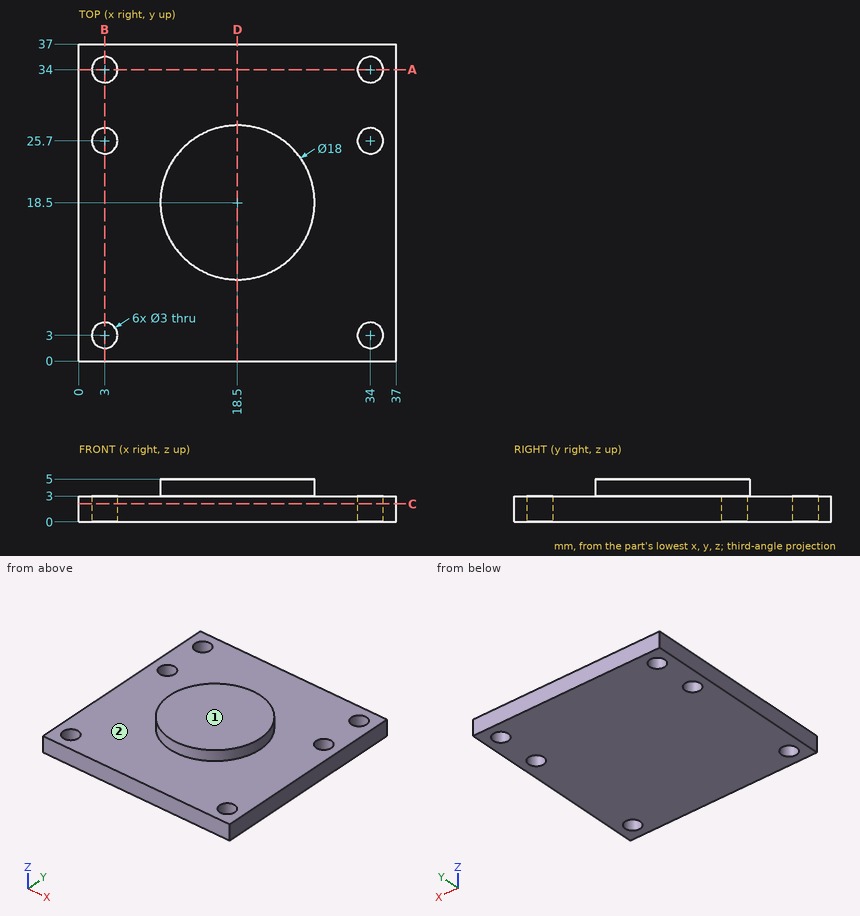
The drawing under review shows one solid part. Ordinate dimensions are in mm from its lowest x, y, z. A direction names the side the tool comes from. Round coordinates to 2 decimals unless told otherwise and drop trailing zeros. Loops run counter-clockwise (first coordinate to the right, second up) from the corner with the lowest first, then second, coordinate; pieces in that order, holes last. Notation, with made-up numbers: (21.25, 53) - (28.25, 53) arc R31 ccw to (28.25, 86) - close; hole circle Ø8 at (36.25, 5). An arc over 180 degrees is marked (long way). One line per item, written item: value. Start each with the question number.
1) Consider section C-C on z = 2.1. Give the boundary of the cut face in (x, y).
2) Consider section D-D on x = 18.5. Give the boundary of the cut face in (y, z).
3) Consider section B-B on x = 3. Give the boundary of the cut face in (y, z).
4) For the marked faces 1 and 2, list the 3-axis set-ups (+Z, -Z, +X, -X, +Y, -Y) from which the entire face can be reached by the end or side of a thin tool; tool diameter is ignored.
5) Insertion check: pin 1 Ø5 at (x, y) = (34, 25.7) entering from +Z; pin 2 Ø2 at (y, z) = (10.5, 4.5) entering from -X. Each pin has a flat end and moves straight along its axis. Give the tip position at first contact, or say it passes through.
6) To check wall thickness, follow L1, parallel to Y at x = 3, z = 1.6; L2, parallel to Z at x = 7.5, y = 32; L3, parallel to Y at x = 16.5, z = 3.05. State the ranges of each line that lie inside material, in increasing order. Write a range as from..to.
7) Consider section A-A on y = 34. Give the boundary of the cut face in (x, z).
Reported:
1. outline: (0, 0) - (37, 0) - (37, 37) - (0, 37) - close; hole circle Ø3 at (3, 3); hole circle Ø3 at (3, 25.7); hole circle Ø3 at (3, 34); hole circle Ø3 at (34, 3); hole circle Ø3 at (34, 25.7); hole circle Ø3 at (34, 34)
2. outline: (0, 0) - (37, 0) - (37, 3) - (27.5, 3) - (27.5, 5) - (9.5, 5) - (9.5, 3) - (0, 3) - close
3. outline: (0, 0) - (1.5, 0) - (1.5, 3) - (0, 3) - close; (4.5, 0) - (24.2, 0) - (24.2, 3) - (4.5, 3) - close; (27.2, 0) - (32.5, 0) - (32.5, 3) - (27.2, 3) - close; (35.5, 0) - (37, 0) - (37, 3) - (35.5, 3) - close
4. face 1: +Z, +X, -X, +Y, -Y
4. face 2: +Z
5. pin 1: stops at z = 3
5. pin 2: stops at x = 12.84
6. L1: y = 0..1.5, 4.5..24.2, 27.2..32.5, 35.5..37
6. L2: z = 0..3
6. L3: y = 9.73..27.27
7. outline: (0, 0) - (1.5, 0) - (1.5, 3) - (0, 3) - close; (4.5, 0) - (32.5, 0) - (32.5, 3) - (4.5, 3) - close; (35.5, 0) - (37, 0) - (37, 3) - (35.5, 3) - close
